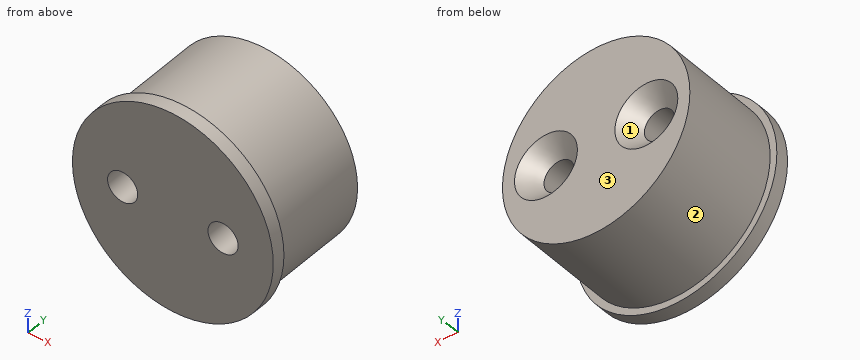
```python
from build123d import *

# Parameters (mm, degrees)
HOLE_WIZARD_M4_1_D           = 4.5
HOLE_WIZARD_M4_1_DEPTH       = 17
HOLE_WIZARD_M4_1_CSINK_D     = 9.4
HOLE_WIZARD_M4_1_CSINK_ANGLE = 90


with BuildPart() as part:
    # 스케치1 → 회전1 (revolve)
    with BuildSketch(Plane.XY):
        Polygon((0, 0), (-15, 0), (-15, 2), (-14, 2), (-14, 17), (0, 17), align=None)
    revolve(axis=Axis((0, 0, 0), (0, 1, 0)))

    # M4 접시 머리 나사용 카운터싱크1
    with Locations(Plane(origin=(0, 17, 0), x_dir=(1, 0, 0), z_dir=(0, 1, 0))):
        with Locations((-7.5, 0), (7.5, 0)):
            CounterSinkHole(HOLE_WIZARD_M4_1_D / 2, HOLE_WIZARD_M4_1_CSINK_D / 2, depth=HOLE_WIZARD_M4_1_DEPTH, counter_sink_angle=HOLE_WIZARD_M4_1_CSINK_ANGLE)


solid = part.part
```
Here's how the part is built. I have some questions about the finished solid (model axes, mm). Face numbers are marked on the shaded views. Round coordinates to 2 decimals unless told otherwise and drop trailing zeros. Order: outer loops, then holes, each group sorted by start corner. A loop starts at its lowest first (then second) coordinate and runs counter-clockwise, first axis right, second up. Notation, with made-up numbers: M 53,-21 L 96,-21 A26 ccw 96,-2 Z; hole C 21.25,59.25 d8. An arc over 180 degrees is marked long. Use CSV: the item, a comma, the result in double quotes.
1) I want a section at C-C (x = -7.5). List the corners of the cut face in (y, z) for me, then the cut area to 3 significant figures.
Taken from the geometry:
outline,"M 0,-12.99 L 2,-12.99 L 2,-11.82 L 17,-11.82 L 17,-4.7 L 14.55,-2.25 L 0,-2.25 Z; M 0,2.25 L 14.55,2.25 L 17,4.7 L 17,11.82 L 2,11.82 L 2,12.99 L 0,12.99 Z"
area,"324 mm^2"
2) If we mould it in two halves opening along X, with no side actions, what happens to the marked faces 1, 2 and 3? For each: pulls with the +X half, pulls with the -X half, needs draft (parallel to the pull), parting line crosses it, or undercut.
Taken from the geometry:
face 1,"undercut"
face 2,"parting line crosses it"
face 3,"needs draft"
3) I want a section at A-A (z = 0). List the corners of the cut face in (x, y) for me.
Taken from the geometry:
outline,"M -15,0 L -9.75,0 L -9.75,14.55 L -12.2,17 L -14,17 L -14,2 L -15,2 Z; M -5.25,0 L 5.25,0 L 5.25,14.55 L 2.8,17 L -2.8,17 L -5.25,14.55 Z; M 9.75,0 L 15,0 L 15,2 L 14,2 L 14,17 L 12.2,17 L 9.75,14.55 Z"
4) I need wall thicknesses on line 1 along X through (y, z) = (4.5, 1.25); line 2 along Z through (x, y) = (5.5, 10); line 3 along Z through (x, y) = (7.5, 4). Which ranges of each line are inside material? Lowest first, please. Write a range as [from, to].
Taken from the geometry:
line 1,"[-13.94, -9.37], [-5.63, 5.63], [9.37, 13.94]"
line 2,"[-12.87, -1.03], [1.03, 12.87]"
line 3,"[-11.82, -2.25], [2.25, 11.82]"
5) I want a section at D-D (y = 12.5). List the corners of the cut face in (x, z) for me.
Taken from the geometry:
outline,"C 0,0 d28; hole C -7.5,0 d4.5; hole C 7.5,0 d4.5"
6) I want a section at B-B (x = 0). List the corners of the cut face in (y, z) for me.
Taken from the geometry:
outline,"M 0,-15 L 2,-15 L 2,-14 L 17,-14 L 17,14 L 2,14 L 2,15 L 0,15 Z"
7) I'm going to push flat-ended pins straight in: P1, Ø1, axis at y = 3, z = 1.5, coming from the -X side; P2, Ø1, axis at x = -3.5, y = 11.5, coming from the +Z side; P3, Ø1.5, axis at x = 4, z = 1, coming from the +Y side. Where does each tip first touch, or does it pass through?
Taken from the geometry:
P1,"x = -13.96"
P2,"z = 13.67"
P3,"y = 16.69"
